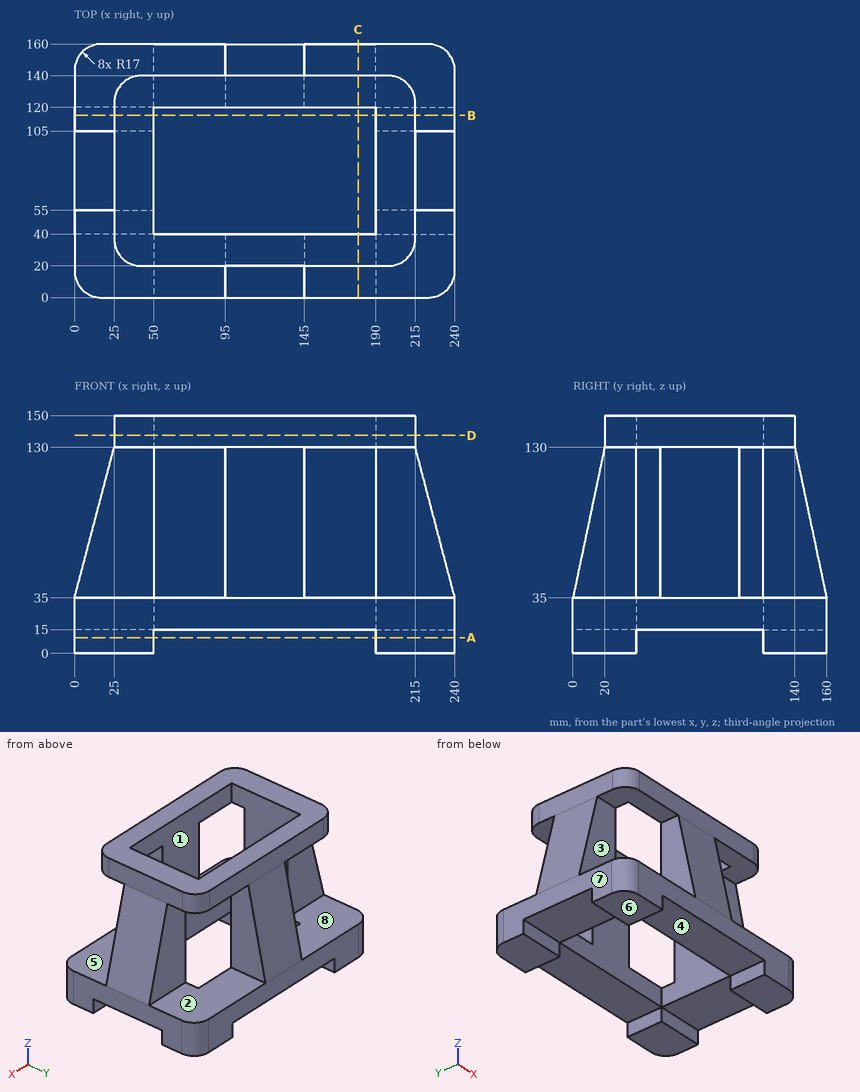
Drawing for the job (mm, zero at the part's lowest x, y, z). A direction names the side the tool comes from. Give positions to 0.01 mm unless a question says otherwise; leave off trailing zeros. Write each loop counter-clockwise with the first axis right and the second up, starting at its lowest first coordinate (ties: lowest second). Pieces come first, ordered by that corner, then holes. Notation, with made-up numbers: (49, 14.25) -> (78, 14.25) arc R9 ccw to (78, 24.25) -> close; hole circle Ø7 at (77.5, -23.75). An arc over 180 degrees is marked (long way). Put each result on its own line as item: value. Start each with the question number.
Item 1: Cut at B-B (y = 115). List the corners of the cut face in (x, z), then the cut area to 3 significant figures.
Item 2: Cut at D-D (z = 137.5). List the corners of the cut face in (x, y).
Item 3: Pin check, flat tips, straight feed: pin 1 Ø22 at (y, z) = (66, 143.5) entering from +X; pin 2 Ø5 at (x, y) = (57, 27.5) entering from -Z; pin 3 Ø22 at (x, z) = (130.5, 144) entering from +Y. Stop position of each tip, or through.
Item 4: Which spindle directions (+Z, -Z, +X, -X, +Y, -Y) get a long thin tool onto all of the face, cutting with end or side? Do the marked faces 1, 2, 3, 4 and 5. Say none if no direction does.
Item 5: Cut at C-C (x = 179). List the corners of the cut face in (y, z), then the cut area to 3 significant figures.
Item 6: Cut at A-A (z = 10). List the corners of the cut face in (x, y), then the cut area to 3 significant figures.
Item 7: Pull direction Z, two halves, no side cores. Call the marked faces 6, 7 and 8: pulls with the +Z half, pulls with the -Z half, needs draft (parallel to the pull), parting line crosses it, or undercut.
Item 8: Wall check: L1, parallel to Z at x = 78, y = 37.5; L2, parallel to Y at x = 69, z = 141; L3, parallel to X at y = 102, z = 141. Give the ranges that are in metal, low to high. Write a range as [from, to].
Answer list:
1. outline: (0, 15) -> (50, 15) -> (50, 35) -> (0, 35) -> close; (25, 130) -> (50, 130) -> (50, 150) -> (25, 150) -> close; (190, 15) -> (240, 15) -> (240, 35) -> (190, 35) -> close; (190, 130) -> (215, 130) -> (215, 150) -> (190, 150) -> close
1. area: 3,000 mm2
2. outline: (25, 37) arc R17 ccw to (42, 20) -> (198, 20) arc R17 ccw to (215, 37) -> (215, 123) arc R17 ccw to (198, 140) -> (42, 140) arc R17 ccw to (25, 123) -> close; hole (50, 40) -> (190, 40) -> (190, 120) -> (50, 120) -> close
3. pin 1: stops at x = 215
3. pin 2: stops at z = 15
3. pin 3: stops at y = 140
4. face 1: +Z, -Z
4. face 2: +X, +Y
4. face 3: +X, -X, -Y
4. face 4: -Z, +Y, -Y
4. face 5: +X, -Y
5. outline: (0, 15) -> (40, 15) -> (40, 35) -> (0, 35) -> close; (20, 130) -> (40, 130) -> (40, 150) -> (20, 150) -> close; (120, 15) -> (160, 15) -> (160, 35) -> (120, 35) -> close; (120, 130) -> (140, 130) -> (140, 150) -> (120, 150) -> close
5. area: 2,400 mm2
6. outline: (0, 17) arc R17 ccw to (17, 0) -> (50, 0) -> (50, 40) -> (0, 40) -> close; (0, 120) -> (50, 120) -> (50, 160) -> (17, 160) arc R17 ccw to (0, 143) -> close; (190, 0) -> (223, 0) arc R17 ccw to (240, 17) -> (240, 40) -> (190, 40) -> close; (190, 120) -> (240, 120) -> (240, 143) arc R17 ccw to (223, 160) -> (190, 160) -> close
6. area: 7,750 mm2
7. face 6: pulls with the -Z half
7. face 7: needs draft
7. face 8: undercut
8. L1: z = [15, 35], [130, 150]
8. L2: y = [20, 40], [120, 140]
8. L3: x = [25, 50], [190, 215]
